Part model, mm, in its own coordinate system. A direction names the side the tool comes from. Round coordinates to 2 decimals unless told otherwise and drop trailing zeros. Write each loop counter-clockwise with the first axis right and the second up, starting at its lowest first coordinate (ties: lowest second). Pieces come first, ordered by that corner, then holes.
```python
from build123d import *

# Parameters (mm, degrees)
BOSS_EXTRUDE1_DEPTH            = 63.5
BOSS_EXTRUDE1_DEPTH_BACK       = 63.5
SKETCH1_W                      = 76.2
SKETCH1_H                      = 76.2
SKETCH1_W_2                    = 63.5
SKETCH1_H_2                    = 63.5
F_4_40_TAPPED_HOLE1_AT_2_COUNT = 2
F_4_40_TAPPED_HOLE1_AT_2_PITCH = 69.85
F_4_40_TAPPED_HOLE1_AT_3_COUNT = 2
F_4_40_TAPPED_HOLE1_AT_3_PITCH = 98.782817332
F_4_40_TAPPED_HOLE1_AT_4_COUNT = 2
F_4_40_TAPPED_HOLE1_AT_4_PITCH = 69.85
CBORE_FOR_M3_SHCS1_D           = 3.4
CBORE_FOR_M3_SHCS1_DEPTH       = 6.35
CBORE_FOR_M3_SHCS1_CBORE_D     = 6.5
CBORE_FOR_M3_SHCS1_CBORE_DEPTH = 3


with BuildPart() as part:
    # Sketch1 → Boss-Extrude1 (new, two sides: drawn at the far end of the back side and taken through both)
    with BuildSketch(Plane(origin=(0, 0, 0), x_dir=(0, 0, -1), z_dir=(1, 0, 0)).offset(-BOSS_EXTRUDE1_DEPTH_BACK)):
        Rectangle(SKETCH1_W, SKETCH1_H)
        Rectangle(SKETCH1_W_2, SKETCH1_H_2, mode=Mode.SUBTRACT)
    extrude(amount=BOSS_EXTRUDE1_DEPTH + BOSS_EXTRUDE1_DEPTH_BACK)

    # Sketch3 → #4-40 Tapped Hole1 (revolve, cut)
    with BuildSketch(Plane(origin=(63.5, 34.925, 34.925), x_dir=(0, 0, -1), z_dir=(0, 1, 0))):
        Polygon((0, 0), (0, 8.299152758), (1.1303, 7.62), (1.1303, 0), align=None)
    f_4_40_tapped_hole1 = revolve(axis=Axis((69.85, 34.925, 34.925), (-1, 0, 0)), mode=Mode.SUBTRACT)

    # #4-40 Tapped Hole1 at 2: #4-40 Tapped Hole1 ×2
    with Locations(*[(0, 0, -i * F_4_40_TAPPED_HOLE1_AT_2_PITCH) for i in range(1, F_4_40_TAPPED_HOLE1_AT_2_COUNT)]):
        add(f_4_40_tapped_hole1, mode=Mode.SUBTRACT)

    # #4-40 Tapped Hole1 at 3: #4-40 Tapped Hole1 ×2
    with Locations(*[Vector(0, -0.7071067811865475, -0.7071067811865476) * (i * F_4_40_TAPPED_HOLE1_AT_3_PITCH) for i in range(1, F_4_40_TAPPED_HOLE1_AT_3_COUNT)]):
        add(f_4_40_tapped_hole1, mode=Mode.SUBTRACT)

    # #4-40 Tapped Hole1 at 4: #4-40 Tapped Hole1 ×2
    with Locations(*[(0, -i * F_4_40_TAPPED_HOLE1_AT_4_PITCH, 0) for i in range(1, F_4_40_TAPPED_HOLE1_AT_4_COUNT)]):
        add(f_4_40_tapped_hole1, mode=Mode.SUBTRACT)

    # Mirror1: #4-40 Tapped Hole1 across plane
    add(f_4_40_tapped_hole1.mirror(Plane(origin=(0, 0, 0), x_dir=(0, 0, 1), z_dir=(1, 0, 0))), mode=Mode.SUBTRACT)

    # Mirror1 copy 1 sketch → Mirror1 copy 1 (revolve, cut)
    with BuildSketch(Plane(origin=(-63.5, 34.925, -34.925), x_dir=(0, 0, -1), z_dir=(0, 1, 0))):
        Polygon((0, 0), (0, -8.299152758), (1.1303, -7.62), (1.1303, 0), align=None)
    revolve(axis=Axis((-69.85, 34.925, -34.925), (-1, 0, 0)), mode=Mode.SUBTRACT)

    # Mirror1 copy 2 sketch → Mirror1 copy 2 (revolve, cut)
    with BuildSketch(Plane(origin=(-63.5, -34.925, -34.925), x_dir=(0, 0, -1), z_dir=(0, 1, 0))):
        Polygon((0, 0), (0, -8.299152758), (1.1303, -7.62), (1.1303, 0), align=None)
    revolve(axis=Axis((-69.85, -34.925, -34.925), (-1, 0, 0)), mode=Mode.SUBTRACT)

    # Mirror1 copy 3 sketch → Mirror1 copy 3 (revolve, cut)
    with BuildSketch(Plane(origin=(-63.5, -34.925, 34.925), x_dir=(0, 0, -1), z_dir=(0, 1, 0))):
        Polygon((0, 0), (0, -8.299152758), (1.1303, -7.62), (1.1303, 0), align=None)
    revolve(axis=Axis((-69.85, -34.925, 34.925), (-1, 0, 0)), mode=Mode.SUBTRACT)

    # CBORE for M3 SHCS1
    with Locations(Plane(origin=(0, -38.1, 0), x_dir=(-1, 0, 0), z_dir=(0, -1, 0))):
        with Locations((-52.09999994, 19.499999922), (-12.7, 19.499999922), (-12.7, -19.900000078), (-52.1, -19.900000078)):
            CounterBoreHole(CBORE_FOR_M3_SHCS1_D / 2, CBORE_FOR_M3_SHCS1_CBORE_D / 2, CBORE_FOR_M3_SHCS1_CBORE_DEPTH, depth=CBORE_FOR_M3_SHCS1_DEPTH)


solid = part.part
```
Q1. Cut at A-A on z = -13. Write the cut outline in (x, y).
Values follow:
outline: (-63.5, -38.1) - (63.5, -38.1) - (63.5, -31.75) - (-63.5, -31.75) - close; (-63.5, 31.75) - (63.5, 31.75) - (63.5, 38.1) - (-63.5, 38.1) - close
Q2. Mould opens along Y. For faces 1 (the cylindrical face through (12.33, -33.4, -17.84)), 2 (the flat face through (-1, 0, -31.75)), 3 (the flat face through (-1, -38.1, 1)) say: +Y half, -Y half, draft (parallel to the pull), parting line (faces both ways), or undercut.
Values follow:
face 1: draft
face 2: undercut
face 3: -Y half
Q3. Wall check: L1, parallel to Z at x = 52.1, y = -36.2; L2, parallel to Y at x = -2, z = 11. Give the ranges that are in metal, low to high.
Values follow:
L1: z = -38.1 to -22.75, -16.25 to 16.65, 23.15 to 38.1
L2: y = -38.1 to -31.75, 31.75 to 38.1
Q4. Which spindle directions (+Z, -Z, +X, -X, +Y, -Y) get a long thin tool onto all of the face, cutting with end or side? Do faces 4 (the cylindrical face through (15.947, -36.621, 19.757)), 5 (the flat face through (-1, 31.75, 0)), 6 (the flat face through (-1, 38.1, 1)). Say none if no direction does.
Values follow:
face 4: -Y
face 5: +X, -X
face 6: +Z, -Z, +X, -X, +Y
Q5. Cut at D-D on x = 32.5. Write the cut outline in (y, z), plus the area to 3 significant figures.
Values follow:
outline: (-38.1, -38.1) - (38.1, -38.1) - (38.1, 38.1) - (-38.1, 38.1) - close; hole (-31.75, -31.75) - (31.75, -31.75) - (31.75, 31.75) - (-31.75, 31.75) - close
area: 1,770 mm2
Q6. Drop flat-ended pins along their axis: pin 1 (3.5 mm diameter, centred on y = 34.925, z = 34.925, fed in from -X); pin 2 (2 mm diameter, centred on y = 34.925, z = -34.925, fed in from -X); pin 3 (3 mm diameter, centred on x = 12.7, z = -19.5, fed in from -Y); pin 4 (6 mm diameter, centred on x = 12.7, z = 19.9, fed in from -Y). Give the stop position or say it passes through.
Values follow:
pin 1: stops at x = -63.5
pin 2: stops at x = -55.8
pin 3: stops at y = 31.75
pin 4: stops at y = -35.1
Q7. Cut at C-C on x = 12.7. Write the cut outline in (y, z).
Values follow:
outline: (-38.1, -38.1) - (38.1, -38.1) - (38.1, 38.1) - (-38.1, 38.1) - (-38.1, 23.15) - (-35.1, 23.15) - (-35.1, 21.6) - (-31.75, 21.6) - (-31.75, 31.75) - (31.75, 31.75) - (31.75, -31.75) - (-31.75, -31.75) - (-31.75, -21.2) - (-35.1, -21.2) - (-35.1, -22.75) - (-38.1, -22.75) - close; (-38.1, -16.25) - (-35.1, -16.25) - (-35.1, -17.8) - (-31.75, -17.8) - (-31.75, 18.2) - (-35.1, 18.2) - (-35.1, 16.65) - (-38.1, 16.65) - close
